Can you work these out from the drawing? Everything is in mm from the part's minimum corner. Coordinates: 2 decimals unless noted, no trailing zeros. Loops run counter-clockwise (first coordinate to the right, second up) from the corner with the lowest first, then second, coordinate; pieces in that order, holes last. Notation, with made-up numbers: M 85,22 L 119,22 A28 cw 119,49 Z; hole C 30.5,-1.5 d4. An arc over 180 degrees is marked long. Write each question's results on one line, items separated by ' | '.
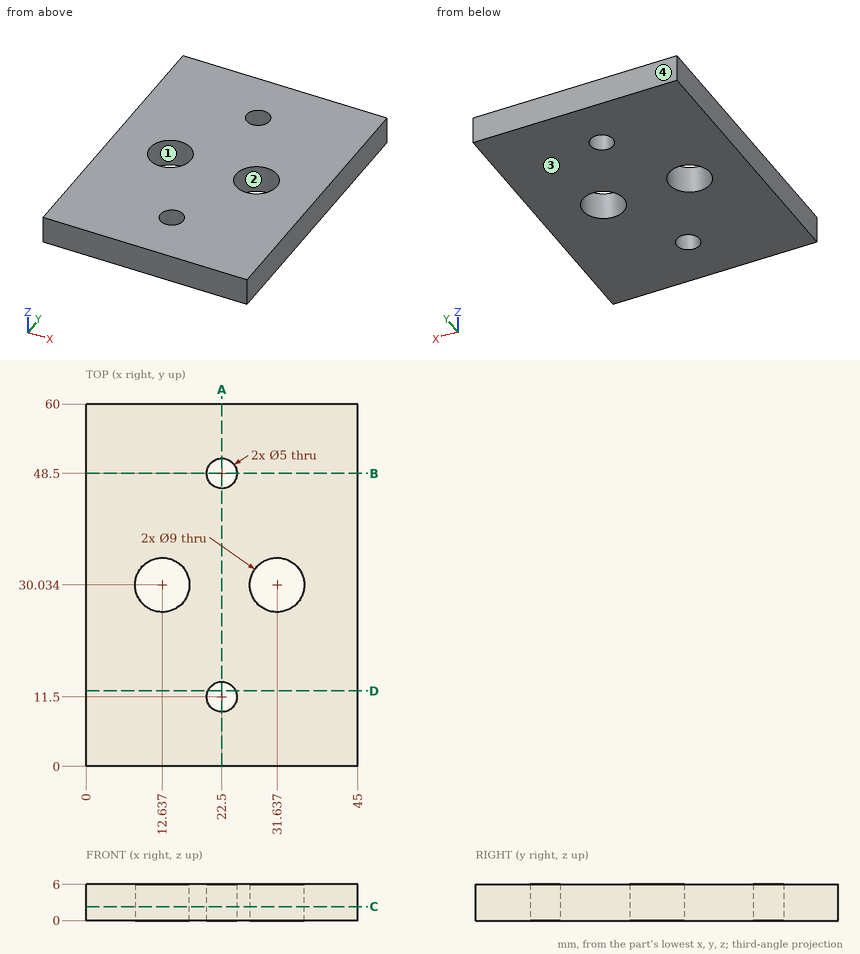
(1) Imagine slicing it at A-A, the plane x = 22.5. List the corners of the cut face in (y, z) for me.
Reported:
outline: M 0,0 L 9,0 L 9,6 L 0,6 Z; M 14,0 L 46,0 L 46,6 L 14,6 Z; M 51,0 L 60,0 L 60,6 L 51,6 Z
(2) Please list where these lines run through material, in increasing order: probe 1 along Y at (x, z) = (22.5, 1.45); probe 2 along X at (y, z) = (33.5, 4.6); probe 3 along X at (y, z) = (29.5, 3.6) (1 decimal). Write a range as from..to.
Reported:
probe 1: y = 0..9, 14..46, 51..60 | probe 2: x = 0..9.77, 15.51..28.77, 34.51..45 | probe 3: x = 0..8.2, 17.1..27.2, 36.1..45
(3) Imagine slicing it at B-B, the plane y = 48.5. List the corners of the cut face in (x, z) for me.
Reported:
outline: M 0,0 L 20,0 L 20,6 L 0,6 Z; M 25,0 L 45,0 L 45,6 L 25,6 Z
(4) If we mould it in two halves opening along Y, with no side actions, what happens to the marked faces 1, 2, 3 and 4? For each: released by +Y, released by -Y, zero draft, split by the parting line, or undercut.
Reported:
face 1: undercut | face 2: undercut | face 3: zero draft | face 4: released by +Y
(5) Imagine slicing it at D-D, the plane y = 12.5. List the corners of the cut face in (x, z) for me, and give its area (4 significant figures).
Reported:
outline: M 0,0 L 20.21,0 L 20.21,6 L 0,6 Z; M 24.79,0 L 45,0 L 45,6 L 24.79,6 Z | area: 242.5 mm2
(6) Will this pin go through, and if not, where does the flat tip stop? P1, Ø8, axis at x = 12.64, y = 30.03, coming from the -Z side.
Reported:
P1: passes through
(7) Imagine slicing it at C-C, the plane z = 2.3. List the corners of the cut face in (x, y) for me, and give its area (3 significant figures).
Reported:
outline: M 0,0 L 45,0 L 45,60 L 0,60 Z; hole C 12.64,30.03 d9; hole C 22.5,11.5 d5; hole C 22.5,48.5 d5; hole C 31.64,30.03 d9 | area: 2,530 mm2
